Part model, mm, in its own coordinate system. A direction names the side the tool comes from. Round coordinates to 2 decimals unless told otherwise and drop trailing zeros. Loops run counter-clockwise (first coordinate to the right, second up) from the corner with the lowest first, then second, coordinate; pieces in that order, holes last.
from build123d import *

# Parameters (mm, degrees)
SKETCH1_W           = 300
SKETCH1_H           = 220
BOSS_EXTRUDE1_DEPTH = 3
SKETCH2_R           = 12.5
CUT_EXTRUDE1_DEPTH  = 3
SKETCH3_R           = 60
SKETCH3_R_2         = 55
SKETCH3_R_3         = 35
SKETCH3_R_4         = 30
BOSS_EXTRUDE2_DEPTH = 3
CUT_EXTRUDE2_REACH  = 188.107
SKETCH4_R           = 1.1
CUT_EXTRUDE3_REACH  = 188.035
SKETCH5_R           = 10
SKETCH6_W           = 300
SKETCH6_H           = 30
BOSS_EXTRUDE3_DEPTH = 3
CUT_EXTRUDE4_REACH  = 207.205
SKETCH7_R           = 2.1
CUT_EXTRUDE5_REACH  = 207.205
CUT_EXTRUDE6_REACH  = 207.205
SKETCH10_R          = 4
SKETCH10_R_2        = 9


with BuildPart() as part:
    # Sketch1 → Boss-Extrude1 (new body)
    with BuildSketch(Plane(origin=(0, 0, 0), x_dir=(1, 0, 0), z_dir=(0, 1, 0))):
        Rectangle(SKETCH1_W, SKETCH1_H)
    extrude(amount=BOSS_EXTRUDE1_DEPTH)

    # Sketch2 → Cut-Extrude1 (cut)
    with BuildSketch(Plane(origin=(0, 3, 0), x_dir=(1, 0, 0), z_dir=(0, 1, 0))):
        with Locations(Location((0, 0, 0), (0, 0, 270))):
            Circle(SKETCH2_R)
    extrude(amount=-CUT_EXTRUDE1_DEPTH, mode=Mode.SUBTRACT)

    # Sketch3 → Boss-Extrude2 (add)
    # profile 1 of 2: a face of its own
    with BuildSketch(Plane(origin=(0, 3, 0), x_dir=(1, 0, 0), z_dir=(0, 1, 0))):
        with Locations(Location((0, 0, 0), (0, 0, 270))):
            Circle(SKETCH3_R)
        with Locations(Location((0, 0, 0), (0, 0, 270))):
            Circle(SKETCH3_R_2, mode=Mode.SUBTRACT)
    # profile 2 of 2: a face of its own
    with BuildSketch(Plane(origin=(0, 3, 0), x_dir=(1, 0, 0), z_dir=(0, 1, 0))):
        with Locations(Location((0, 0, 0), (0, 0, 270))):
            Circle(SKETCH3_R_3)
        with Locations(Location((0, 0, 0), (0, 0, 270))):
            Circle(SKETCH3_R_4, mode=Mode.SUBTRACT)
    extrude(amount=BOSS_EXTRUDE2_DEPTH)

    # Sketch4 → Cut-Extrude2 (cut, up to next)
    with BuildSketch(Plane.XZ, mode=Mode.PRIVATE) as cut_extrude2_sk1:
        with Locations(Location((-20.991491193, 7, 0), (0, 0, 270))):
            Circle(SKETCH4_R)
    cut_extrude2_tool1 = extrude(cut_extrude2_sk1.sketch, amount=-CUT_EXTRUDE2_REACH, mode=Mode.PRIVATE) & part.part
    # Sketch4 → Cut-Extrude2 (cut, up to next)
    with BuildSketch(Plane.XZ, mode=Mode.PRIVATE) as cut_extrude2_sk2:
        with Locations(Location((-27.991491193, 0, 0), (0, 0, 270))):
            Circle(SKETCH4_R)
    cut_extrude2_tool2 = extrude(cut_extrude2_sk2.sketch, amount=-CUT_EXTRUDE2_REACH, mode=Mode.PRIVATE) & part.part
    # Sketch4 → Cut-Extrude2 (cut, up to next)
    with BuildSketch(Plane.XZ, mode=Mode.PRIVATE) as cut_extrude2_sk3:
        with Locations(Location((-20.991491193, -7, 0), (0, 0, 270))):
            Circle(SKETCH4_R)
    cut_extrude2_tool3 = extrude(cut_extrude2_sk3.sketch, amount=-CUT_EXTRUDE2_REACH, mode=Mode.PRIVATE) & part.part
    add(cut_extrude2_tool1.solids().sort_by_distance((-20.991491, 0, 7))[0], mode=Mode.SUBTRACT)
    add(cut_extrude2_tool2.solids().sort_by_distance((-27.991491, 0, 0))[0], mode=Mode.SUBTRACT)
    add(cut_extrude2_tool3.solids().sort_by_distance((-20.991491, 0, -7))[0], mode=Mode.SUBTRACT)

    # Sketch5 → Cut-Extrude3 (cut, up to next)
    with BuildSketch(Plane(origin=(0, 3, 0), x_dir=(1, 0, 0), z_dir=(0, 1, 0)), mode=Mode.PRIVATE) as cut_extrude3_sk1:
        with Locations(Location((0, 75, 0), (0, 0, 270))):
            Circle(SKETCH5_R)
    cut_extrude3_tool1 = extrude(cut_extrude3_sk1.sketch, amount=-CUT_EXTRUDE3_REACH, mode=Mode.PRIVATE) & part.part
    add(cut_extrude3_tool1.solids().sort_by_distance((0, 3, -75))[0], mode=Mode.SUBTRACT)

    # Sketch6 → Boss-Extrude3 (add)
    with BuildSketch(Plane(origin=(0, 3, 0), x_dir=(1, 0, 0), z_dir=(0, 1, 0))):
        with Locations((0, -125)):
            Rectangle(SKETCH6_W, SKETCH6_H)
    extrude(amount=-BOSS_EXTRUDE3_DEPTH)

    # Sketch7 → Cut-Extrude4 (cut, up to next)
    with BuildSketch(Plane(origin=(0, 3, 0), x_dir=(1, 0, 0), z_dir=(0, 1, 0)), mode=Mode.PRIVATE) as cut_extrude4_sk1:
        with Locations(Location((-142, 102, 0), (0, 0, 270))):
            Circle(SKETCH7_R)
    cut_extrude4_tool1 = extrude(cut_extrude4_sk1.sketch, amount=-CUT_EXTRUDE4_REACH, mode=Mode.PRIVATE) & part.part
    # Sketch7 → Cut-Extrude4 (cut, up to next)
    with BuildSketch(Plane(origin=(0, 3, 0), x_dir=(1, 0, 0), z_dir=(0, 1, 0)), mode=Mode.PRIVATE) as cut_extrude4_sk2:
        with Locations(Location((142, 102, 0), (0, 0, 270))):
            Circle(SKETCH7_R)
    cut_extrude4_tool2 = extrude(cut_extrude4_sk2.sketch, amount=-CUT_EXTRUDE4_REACH, mode=Mode.PRIVATE) & part.part
    # Sketch7 → Cut-Extrude4 (cut, up to next)
    with BuildSketch(Plane(origin=(0, 3, 0), x_dir=(1, 0, 0), z_dir=(0, 1, 0)), mode=Mode.PRIVATE) as cut_extrude4_sk3:
        with Locations(Location((142, -132, 0), (0, 0, 270))):
            Circle(SKETCH7_R)
    cut_extrude4_tool3 = extrude(cut_extrude4_sk3.sketch, amount=-CUT_EXTRUDE4_REACH, mode=Mode.PRIVATE) & part.part
    # Sketch7 → Cut-Extrude4 (cut, up to next)
    with BuildSketch(Plane(origin=(0, 3, 0), x_dir=(1, 0, 0), z_dir=(0, 1, 0)), mode=Mode.PRIVATE) as cut_extrude4_sk4:
        with Locations(Location((-142, -132, 0), (0, 0, 270))):
            Circle(SKETCH7_R)
    cut_extrude4_tool4 = extrude(cut_extrude4_sk4.sketch, amount=-CUT_EXTRUDE4_REACH, mode=Mode.PRIVATE) & part.part
    add(cut_extrude4_tool1.solids().sort_by_distance((-142, 3, -102))[0], mode=Mode.SUBTRACT)
    add(cut_extrude4_tool2.solids().sort_by_distance((142, 3, -102))[0], mode=Mode.SUBTRACT)
    add(cut_extrude4_tool3.solids().sort_by_distance((142, 3, 132))[0], mode=Mode.SUBTRACT)
    add(cut_extrude4_tool4.solids().sort_by_distance((-142, 3, 132))[0], mode=Mode.SUBTRACT)

    # Sketch9 → Cut-Extrude5 (cut, up to next)
    with BuildSketch(Plane(origin=(0, 3, 0), x_dir=(1, 0, 0), z_dir=(0, 1, 0)), mode=Mode.PRIVATE) as cut_extrude5_sk1:
        with BuildLine():
            Line((75.252149951, -67.516466644), (72.271396026, -70.624077628))
            ThreePointArc((72.271396026, -70.624077628), (68.544792703, -70.701725066), (68.467145265, -66.975121742))
            Line((68.467145265, -66.975121742), (71.44789919, -63.867510758))
            ThreePointArc((71.44789919, -63.867510758), (75.174502513, -63.78986332), (75.252149951, -67.516466644))
        make_face()
    cut_extrude5_tool1 = extrude(cut_extrude5_sk1.sketch, amount=-CUT_EXTRUDE5_REACH, mode=Mode.PRIVATE) & part.part
    # Sketch9 → Cut-Extrude5 (cut, up to next)
    with BuildSketch(Plane(origin=(0, 3, 0), x_dir=(1, 0, 0), z_dir=(0, 1, 0)), mode=Mode.PRIVATE) as cut_extrude5_sk2:
        with BuildLine():
            Line((72.232976728, -108.891711148), (75.213730653, -111.872465073))
            ThreePointArc((75.213730653, -111.872465073), (75.213730653, -115.599877238), (71.486318487, -115.599877238))
            Line((71.486318487, -115.599877238), (68.505564562, -112.619123313))
            ThreePointArc((68.505564562, -112.619123313), (68.505564562, -108.891711148), (72.232976728, -108.891711148))
        make_face()
    cut_extrude5_tool2 = extrude(cut_extrude5_sk2.sketch, amount=-CUT_EXTRUDE5_REACH, mode=Mode.PRIVATE) & part.part
    # Sketch9 → Cut-Extrude5 (cut, up to next)
    with BuildSketch(Plane(origin=(0, 3, 0), x_dir=(1, 0, 0), z_dir=(0, 1, 0)), mode=Mode.PRIVATE) as cut_extrude5_sk3:
        with BuildLine():
            Line((120.245775281, -112.587078686), (117.2009321, -115.631921866))
            ThreePointArc((117.2009321, -115.631921866), (113.473519935, -115.631921866), (113.473519935, -111.9045097))
            Line((113.473519935, -111.9045097), (116.518363115, -108.85966652))
            ThreePointArc((116.518363115, -108.85966652), (120.245775281, -108.85966652), (120.245775281, -112.587078686))
        make_face()
    cut_extrude5_tool3 = extrude(cut_extrude5_sk3.sketch, amount=-CUT_EXTRUDE5_REACH, mode=Mode.PRIVATE) & part.part
    # Sketch9 → Cut-Extrude5 (cut, up to next)
    with BuildSketch(Plane(origin=(0, 3, 0), x_dir=(1, 0, 0), z_dir=(0, 1, 0)), mode=Mode.PRIVATE) as cut_extrude5_sk4:
        with BuildLine():
            Line((117.2009321, -63.85966652), (120.245775281, -66.9045097))
            ThreePointArc((120.245775281, -66.9045097), (120.245775281, -70.631921866), (116.518363115, -70.631921866))
            Line((116.518363115, -70.631921866), (113.473519935, -67.587078686))
            ThreePointArc((113.473519935, -67.587078686), (113.473519935, -63.85966652), (117.2009321, -63.85966652))
        make_face()
    cut_extrude5_tool4 = extrude(cut_extrude5_sk4.sketch, amount=-CUT_EXTRUDE5_REACH, mode=Mode.PRIVATE) & part.part
    add(cut_extrude5_tool1.solids().sort_by_distance((71.859648, 3, 67.245794))[0], mode=Mode.SUBTRACT)
    add(cut_extrude5_tool2.solids().sort_by_distance((71.859648, 3, 112.245794))[0], mode=Mode.SUBTRACT)
    add(cut_extrude5_tool3.solids().sort_by_distance((116.859648, 3, 112.245794))[0], mode=Mode.SUBTRACT)
    add(cut_extrude5_tool4.solids().sort_by_distance((116.859648, 3, 67.245794))[0], mode=Mode.SUBTRACT)

    # Sketch10 → Cut-Extrude6 (cut, up to next)
    with BuildSketch(Plane(origin=(0, 3, 0), x_dir=(1, 0, 0), z_dir=(0, 1, 0)), mode=Mode.PRIVATE) as cut_extrude6_sk1:
        with Locations(Location((0, -90, 0), (0, 0, 270))):
            Circle(SKETCH10_R)
    cut_extrude6_tool1 = extrude(cut_extrude6_sk1.sketch, amount=-CUT_EXTRUDE6_REACH, mode=Mode.PRIVATE) & part.part
    # Sketch10 → Cut-Extrude6 (cut, up to next)
    with BuildSketch(Plane(origin=(0, 3, 0), x_dir=(1, 0, 0), z_dir=(0, 1, 0)), mode=Mode.PRIVATE) as cut_extrude6_sk2:
        with Locations(Location((25, -90, 0), (0, 0, 270))):
            Circle(SKETCH10_R_2)
    cut_extrude6_tool2 = extrude(cut_extrude6_sk2.sketch, amount=-CUT_EXTRUDE6_REACH, mode=Mode.PRIVATE) & part.part
    add(cut_extrude6_tool1.solids().sort_by_distance((0, 3, 90))[0], mode=Mode.SUBTRACT)
    add(cut_extrude6_tool2.solids().sort_by_distance((25, 3, 90))[0], mode=Mode.SUBTRACT)


solid = part.part
1) Tool access for faces 1 (the face through (0, 2, -85)), 2 (the face through (13, 3, 0)): list every direction of +Z, -Z, +X, -X, +Y, -Y with a clear straight run to the whole face (end or side of a thin tool).
Values:
face 1: +Y, -Y
face 2: +Y
2) Slice it at A-A, the plane x = 0. Give the number of separate pieces and of enclosed holes in the cut face, then the cut area to 3 significant figures.
Values:
separate pieces: 4
enclosed holes: 0
area: 651 mm2
3) Slice it at C-C, the plane z = 120. Give the cut face in (x, y), then the cut area to 3 significant figures.
Values:
outline: (-150, 0) - (150, 0) - (150, 3) - (-150, 3) - close
area: 900 mm2
4) Slice it at D-D, the plane x = -105. Give the cut face in (y, z), then the cut area to 3 significant figures.
Values:
outline: (0, -110) - (3, -110) - (3, 140) - (0, 140) - close
area: 750 mm2
5) Drop flat-ended pins along their axis: pin 1 Ø1 at (x, z) = (22.5, -36.5) entering from +Y; pin 2 Ø12 at (x, z) = (108.5, 109.5) entering from -Y; pin 3 Ø1 at (y, z) = (4, 32.5) entering from -X. Give the stop position or say it passes through.
Values:
pin 1: stops at y = 3
pin 2: stops at y = 0
pin 3: stops at x = -50.75
6) Mould opens along X. For faces 3 (the face through (2.64, 4.48, -59.94)), 4 (the face through (0, 2, 86)), 5 (the face through (-49, 6, 26)) say: released by +X, released by -X, zero draft, split by the parting line, or undercut.
Values:
face 3: split by the parting line
face 4: undercut
face 5: zero draft
7) Wall check: line 1 along Z through (x, y) = (-1, 4.3); line 2 along Z through (x, y) = (142, 0.6); line 3 along Z through (x, y) = (4, 3.85). Give the ranges that are in metal, low to high.
Values:
line 1: z = -59.99 to -54.99, -34.99 to -29.98, 29.98 to 34.99, 54.99 to 59.99
line 2: z = -110 to -104.1, -99.9 to 129.9, 134.1 to 140
line 3: z = -59.87 to -54.85, -34.77 to -29.73, 29.73 to 34.77, 54.85 to 59.87
